The listing builds one solid part. Answer for the finished solid, in the listing's coordinates (mm). Round coordinates to 2 decimals unless told otherwise and drop trailing zeros. Order: outer loops, then holes, each group sorted by start corner. A loop starts at its lowest first (then second) coordinate and runs counter-clockwise, first axis right, second up. Notation, with made-up numbers: (56, 63.5) -> (83, 63.5) arc R24 cw to (83, 89.5) -> close; hole circle Ø9 at (43, 55.5). An arc over 180 degrees is marked (long way). Answer in a Markdown table with one row per item. Add a question column.
```python
from build123d import *

# Parameters (mm, degrees)
SKETCH1_R           = 1.25
BOSS_EXTRUDE1_DEPTH = 1.6
SKETCH2_R           = 0.835
CUT_EXTRUDE1_DEPTH  = 10


with BuildPart() as part:
    # Sketch1 → Boss-Extrude1 (new body)
    with BuildSketch(Plane.XY):
        with BuildLine():
            Line((15.61, -11.45), (-15.61, -11.45))
            ThreePointArc((-15.61, -11.45), (-17.406051224, -10.706051224), (-18.15, -8.91))
            Line((-18.15, -8.91), (-18.15, 8.91))
            ThreePointArc((-18.15, 8.91), (-17.406051224, 10.706051224), (-15.61, 11.45))
            Line((-15.61, 11.45), (15.61, 11.45))
            ThreePointArc((15.61, 11.45), (17.406051224, 10.706051224), (18.15, 8.91))
            Line((18.15, 8.91), (18.15, -8.91))
            ThreePointArc((18.15, -8.91), (17.406051224, -10.706051224), (15.61, -11.45))
        make_face()
        with Locations((-15.61, 8.91)):
            Circle(SKETCH1_R, mode=Mode.SUBTRACT)
        with Locations((-15.61, -8.91)):
            Circle(SKETCH1_R, mode=Mode.SUBTRACT)
    extrude(amount=BOSS_EXTRUDE1_DEPTH)

    # Sketch2 → Cut-Extrude1 (cut)
    with BuildSketch(Plane.XY.offset(1.6)):
        with Locations((12.4347, -10.18)):
            Circle(SKETCH2_R)
        with Locations((9.8947, -10.18)):
            Circle(SKETCH2_R)
        with Locations((7.3547, -10.18)):
            Circle(SKETCH2_R)
        with Locations((4.8147, -10.18)):
            Circle(SKETCH2_R)
        with Locations((2.2747, -10.18)):
            Circle(SKETCH2_R)
        with Locations((-0.2653, -10.18)):
            Circle(SKETCH2_R)
        with Locations((-2.8053, -10.18)):
            Circle(SKETCH2_R)
        with Locations((-5.3453, -10.18)):
            Circle(SKETCH2_R)
    extrude(amount=-CUT_EXTRUDE1_DEPTH, mode=Mode.SUBTRACT)


solid = part.part
```
Item 1: The part is cut by section B-B, the plane y = -8.5. Give the vertices of the cut face in (x, z), and give its area (3 significant figures).
Item 2: The part is cut by section A-A, the plane z = 0.95. State how many separate pieces and enclosed holes the cut face has, and give its area (3 significant figures).
Item 3: Find the intervals of material crossed by probe 1 along Y at (x, z) = (-15.61, 1.15); probe 2 along Y at (x, z) = (12.5, 1.1); probe 3 along Y at (x, z) = (0, 0.55), in increasing order. Write a range as [from, to].
Item 4: For a pull along X with two mould halves and no side action, classify faces 1 (the face through (17.386, 10.726, 0.789)), 2 (the face through (-17.386, -10.726, 0.789)), 3 (the face through (-4.96, -10.92, 0.81)) as released by +X, released by -X, zero draft, split by the parting line, or undercut.
Item 5: Flat-ended cylindrical pins translate along their axes: P1, Ø2.5, axis at x = -5.35, y = -10.18, coming from the +Z side; P2, Ø1.5, axis at x = -15.61, y = -8.91, coming from the -Z side. Find the tip coordinate at first contact, or state that the pin passes through.
Resolved:
| question | item | result |
|---|---|---|
| 1 | outline | (-18.15, 0) -> (-16.79, 0) -> (-16.79, 1.6) -> (-18.15, 1.6) -> close; (-14.43, 0) -> (18.15, 0) -> (18.15, 1.6) -> (-14.43, 1.6) -> close |
| 1 | area | 54.3 mm2 |
| 2 | separate pieces | 1 |
| 2 | enclosed holes | 10 |
| 2 | area | 798 mm2 |
| 3 | probe 1 | [-11.45, -10.16], [-7.66, 7.66], [10.16, 11.45] |
| 3 | probe 2 | [-11.45, -11.01], [-9.35, 11.45] |
| 3 | probe 3 | [-11.45, -10.97], [-9.39, 11.45] |
| 4 | face 1 | released by +X |
| 4 | face 2 | released by -X |
| 4 | face 3 | undercut |
| 5 | P1 | z = 1.6 |
| 5 | P2 | through |
